CAD build for the part. Positions are in the model's coordinates, mm. Face numbers are marked on the shaded views. Give positions to 0.01 mm unless a question says otherwise; leave off trailing zeros. Order: outer loops, then holes, each group sorted by start corner. A loop starts at its lowest first (then second) coordinate and runs counter-clockwise, first axis right, second up.
Item 1: Band-saw the part on D-D on y = -7. Give the cut face in (x, z), plus the area to 3 significant figures.
Item 2: Wall check: L1, parallel to Y at x = 0, z = 1.9; L2, parallel to Y at x = 1.25, z = 0.3; L3, parallel to Y at x = 7, z = 1.65. Give the ranges that are in metal, low to high.
Item 3: Band-saw the part on C-C on x = -7. Give the cut face in (y, z).
Item 4: Band-saw the part on B-B on x = -0.25. Give the cut face in (y, z), plus the area to 3 significant figures.
Item 5: Band-saw the part on A-A on z = 1.1. Give the cut face in (x, y).
Item 6: Two-plate mould, pull along X, no slides. Class the marked faces 1, 2 and 3: released by +X, released by -X, zero draft, split by the parting line, or undercut.
Item 7: Flat gauge pins, fed straight in: P1, Ø1, axis at y = -8, z = 1, coming from the +X side; P2, Ø2, axis at x = 0, y = -7, coming from the -Z side. Where does each tip first touch, or does it go through?
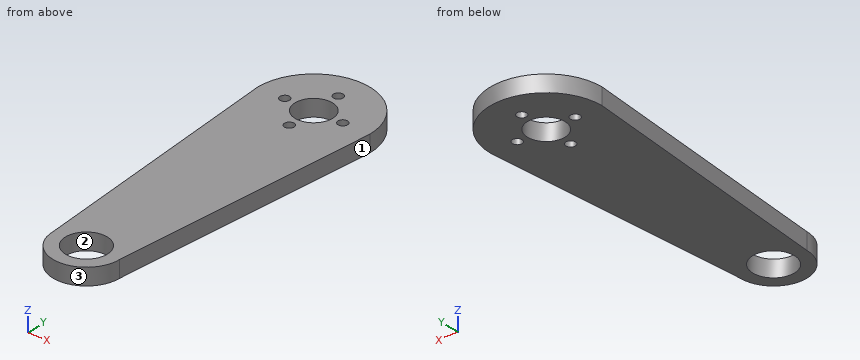
```python
from build123d import *

# Parameters (mm, degrees)
SKETCH_1_R      = 4.5
SKETCH_1_R_2    = 1.15
SKETCH_1_R_3    = 5
EXTRUDE_1_DEPTH = 4


with BuildPart() as part:
    # 草图1 → 凸台-拉伸1 (new body)
    with BuildSketch(Plane.XY):
        with BuildLine():
            Line((-13.5, 0), (-8, -65))
            ThreePointArc((-8, -65), (0, -73), (8, -65))
            Line((8, -65), (13.5, 0))
            ThreePointArc((13.5, 0), (0, 13.5), (-13.5, 0))
        make_face()
        Circle(SKETCH_1_R, mode=Mode.SUBTRACT)
        with Locations((0, 7)):
            Circle(SKETCH_1_R_2, mode=Mode.SUBTRACT)
        with Locations((7, 0)):
            Circle(SKETCH_1_R_2, mode=Mode.SUBTRACT)
        with Locations((0, -7)):
            Circle(SKETCH_1_R_2, mode=Mode.SUBTRACT)
        with Locations((-7, 0)):
            Circle(SKETCH_1_R_2, mode=Mode.SUBTRACT)
        with Locations((0, -65)):
            Circle(SKETCH_1_R_3, mode=Mode.SUBTRACT)
    extrude(amount=EXTRUDE_1_DEPTH)


solid = part.part
```
The answers:
1. outline: (-12.91, 0) - (-1.15, 0) - (-1.15, 4) - (-12.91, 4) - close; (1.15, 0) - (12.91, 0) - (12.91, 4) - (1.15, 4) - close
1. area: 94.1 mm2
2. L1: y = -73 to -70, -60 to -8.15, -5.85 to -4.5, 4.5 to 5.85, 8.15 to 13.5
2. L2: y = -72.9 to -69.84, -60.16 to -4.32, 4.32 to 13.44
2. L3: y = -68.87 to -1.15, 1.15 to 11.54
3. outline: (-68.87, 0) - (-1.15, 0) - (-1.15, 4) - (-68.87, 4) - close; (1.15, 0) - (11.54, 0) - (11.54, 4) - (1.15, 4) - close
4. outline: (-73, 0) - (-69.99, 0) - (-69.99, 4) - (-73, 4) - close; (-60.01, 0) - (-8.12, 0) - (-8.12, 4) - (-60.01, 4) - close; (-5.88, 0) - (-4.49, 0) - (-4.49, 4) - (-5.88, 4) - close; (4.49, 0) - (5.88, 0) - (5.88, 4) - (4.49, 4) - close; (8.12, 0) - (13.5, 0) - (13.5, 4) - (8.12, 4) - close
4. area: 252 mm2
5. outline: (-13.5, 0) - (-8, -65) arc R8 ccw to (8, -65) - (13.5, 0) arc R13.5 ccw to start; hole circle Ø2.3 at (-7, 0); hole circle Ø10 at (0, -65); hole circle Ø9 at (0, 0); hole circle Ø2.3 at (0, -7); hole circle Ø2.3 at (0, 7); hole circle Ø2.3 at (7, 0)
6. face 1: released by +X
6. face 2: undercut
6. face 3: split by the parting line
7. P1: stops at x = 12.87
7. P2: passes through
